from build123d import *

# Parameters (mm, degrees)
F0_R     = 4.75
F1_DEPTH = 7.5
F2_R     = 50
F3_SIZE  = 1
F4_SCALE = 0.62
F6_DEPTH = 25
F7_SIZE  = 0.8


with BuildPart() as f1:
    # F0 (on Top) → F1 (new body, symmetric)
    with BuildSketch(Plane.XY):
        with BuildLine():
            Line((25, 0), (8.2889389183, 39.5062075821))
            ThreePointArc((8.2889389183, 39.5062075821), (0, 45), (-8.2889389183, 39.5062075821))
            Line((-8.2889389183, 39.5062075821), (-25, 0))
            Line((-25, 0), (-8.2889389183, -39.5062075821))
            ThreePointArc((-8.2889389183, -39.5062075821), (0, -45), (8.2889389183, -39.5062075821))
            Line((8.2889389183, -39.5062075821), (25, 0))
        make_face()
        with Locations((0, -36)):
            Circle(F0_R, mode=Mode.SUBTRACT)
        with Locations((0, 36)):
            Circle(F0_R, mode=Mode.SUBTRACT)
    extrude(amount=F1_DEPTH, both=True)

    # F2
    f2_edges = [f1.edges().sort_by_distance(p)[0] for p in [
        (-25, 0, 0),
        (25, 0, 0),
    ]]
    fillet(f2_edges, radius=F2_R)

    # F3
    f3_edges = [f1.edges().sort_by_distance(p)[0] for p in [
        (0, 45, 7.5),
        (0, 45, -7.5),
        (-12.524692, -29.492569, 7.5),
        (-12.524692, -29.492569, -7.5),
    ]]
    chamfer(f3_edges, length=F3_SIZE)


with BuildPart() as f1_1:
    # F4: moved
    add(f1.part.scale(F4_SCALE))

    # F5 (on face) → F6 (cut)
    with BuildSketch(Plane.XY.offset(4.65)):
        Polygon((-2.3094010768, 4), (-4.6188021535, 0), (-2.3094010768, -4), (2.3094010768, -4), (4.6188021535, 0), (2.3094010768, 4), align=None)
    extrude(amount=-F6_DEPTH, mode=Mode.SUBTRACT)

    # F7
    f7_edges = [f1_1.edges().sort_by_distance(p)[0] for p in [
        (0, -4, 4.65),
        (-3.464102, -2, 4.65),
        (-3.464102, 2, 4.65),
        (0, 4, 4.65),
        (3.464102, 2, 4.65),
        (3.464102, -2, 4.65),
        (0, -4, -4.65),
        (3.464102, -2, -4.65),
        (3.464102, 2, -4.65),
        (0, 4, -4.65),
        (-3.464102, 2, -4.65),
        (-2.945, -22.32, 4.65),
        (-2.945, 22.32, 4.65),
        (-2.945, -22.32, -4.65),
        (-2.945, 22.32, -4.65),
    ]]
    chamfer(f7_edges, length=F7_SIZE)


solid = f1_1.part
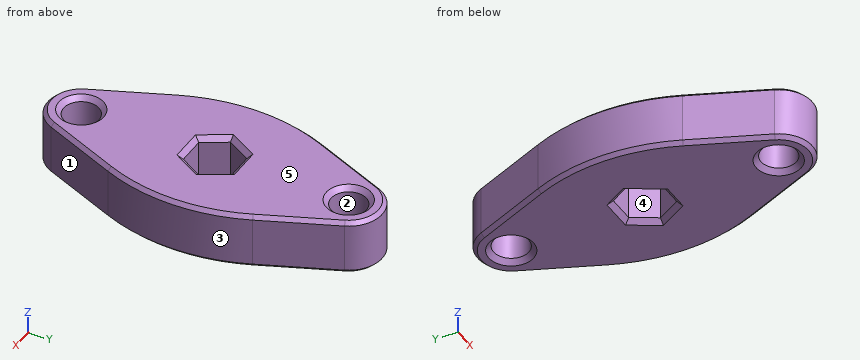
Work out the finished part from the listing and answer in its coordinate system (mm). Face numbers are marked on the shaded views. A direction names the side the tool comes from. Give positions to 0.01 mm unless a question says otherwise; leave off trailing zeros. Write each loop counter-clockwise with the first axis right and the second up, starting at its lowest first coordinate (ties: lowest second). Pieces come first, ordered by that corner, then holes. Notation, with made-up numbers: (3.5, -2) - (31.5, -2) arc R19 cw to (31.5, 25) - close; hole circle Ø9 at (-2.5, -9.5). An arc over 180 degrees is marked (long way). One line per item, written item: value. Start each with the question number.
1. For a pull along Y with two mould halves and no side action, classify the marked faces 1, 2 and 3 as +Y half, -Y half, draft (parallel to the pull), parting line (faces both ways), or undercut.
2. Given pin 1 (3 mm diameter, centred on y = -10, z = -0.5, fed in from +X); pin 2 (1 mm diameter, centred on x = 9.5, y = -16, fed in from +Z); pin 3 (1.5 mm diameter, centred on x = -9, z = 1.5, fed in from +Y); pin 4 (3 mm diameter, centred on y = -11.5, z = 0.5, fed in from -X), each flat-ended and moving along its own axis, determine where each tip first touches the part or whether it passes through.
3. Find section D-D (y = -13). Write down the section's boundary in (x, z).
4. Find section B-B (z = 0.5). Write down the section's boundary in (x, y) (3 decimals), then the cut area to 3 significant figures.
5. Consider probe 1 along Y at (x, z) = (0, 1) (3 decimals); probe 2 along Y at (x, z) = (-1, 0.5); probe 3 along X at (y, z) = (-21, -1). Determine where each line is inside the solid, lowest interval first.
6. For the marked faces 4 and 5, determine the directions among +Z, -Z, +X, -X, +Y, -Y from which every point of the face is accessible in a straight line to the end or side of a thin tool.
7. Find section A-A (x = 0). State how many separate pieces and enclosed holes the cut face has, then the cut area to 3 significant figures.
Geometry results:
1. face 1: -Y half
1. face 2: undercut
1. face 3: parting line
2. pin 1: x = 11.65
2. pin 2: through
2. pin 3: y = 17.14
2. pin 4: x = -11.18
3. outline: (-10, -4.03) - (-9.33, -4.65) - (9.33, -4.65) - (10, -4.03) - (10, 4.03) - (9.33, 4.65) - (-9.33, 4.65) - (-10, 4.03) - close
4. outline: (-10.391, -12.077) - (-5.139, -24.494) arc R5.58 ccw to (5.139, -24.494) - (10.391, -12.077) arc R31 ccw to (10.391, 12.077) - (5.139, 24.494) arc R5.58 ccw to (-5.139, 24.494) - (-10.391, 12.077) arc R31 ccw to start; hole (-4.619, 0) - (-2.309, -4) - (2.309, -4) - (4.619, 0) - (2.309, 4) - (-2.309, 4) - close; hole circle Ø5.89 at (0, -22.32); hole circle Ø5.89 at (0, 22.32)
4. area: 908 mm2
5. probe 1: -27.9 to -25.265, -19.375 to -4, 4 to 19.375, 25.265 to 27.9
5. probe 2: -27.81 to -25.09, -19.55 to -4, 4 to 19.55, 25.09 to 27.81
5. probe 3: -6.62 to -2.63, 2.63 to 6.62
6. face 4: +Z, -Z
6. face 5: +Z, +X, -X, +Y, -Y
7. separate pieces: 4
7. enclosed holes: 0
7. area: 330 mm2
